Answer from the drawing. Dimensions are ordinates in mm from the lowest x, y and z of the part. Coordinates: 2 decimals unless noted, no trailing zeros. Order: outer loops, then holes, each group sorted by start corner. A loop starts at its lowest first (then second) coordinate and runs counter-clockwise, first axis right, second up. Notation, with made-up numbers: (57.25, -37.75) - (61.25, -37.75) arc R21 ccw to (61.25, -9.75) - close; hole circle Ø2 at (-4, 49). An arc over 180 degrees is marked (long way). One line per item, written item: value. Start each with the question number.
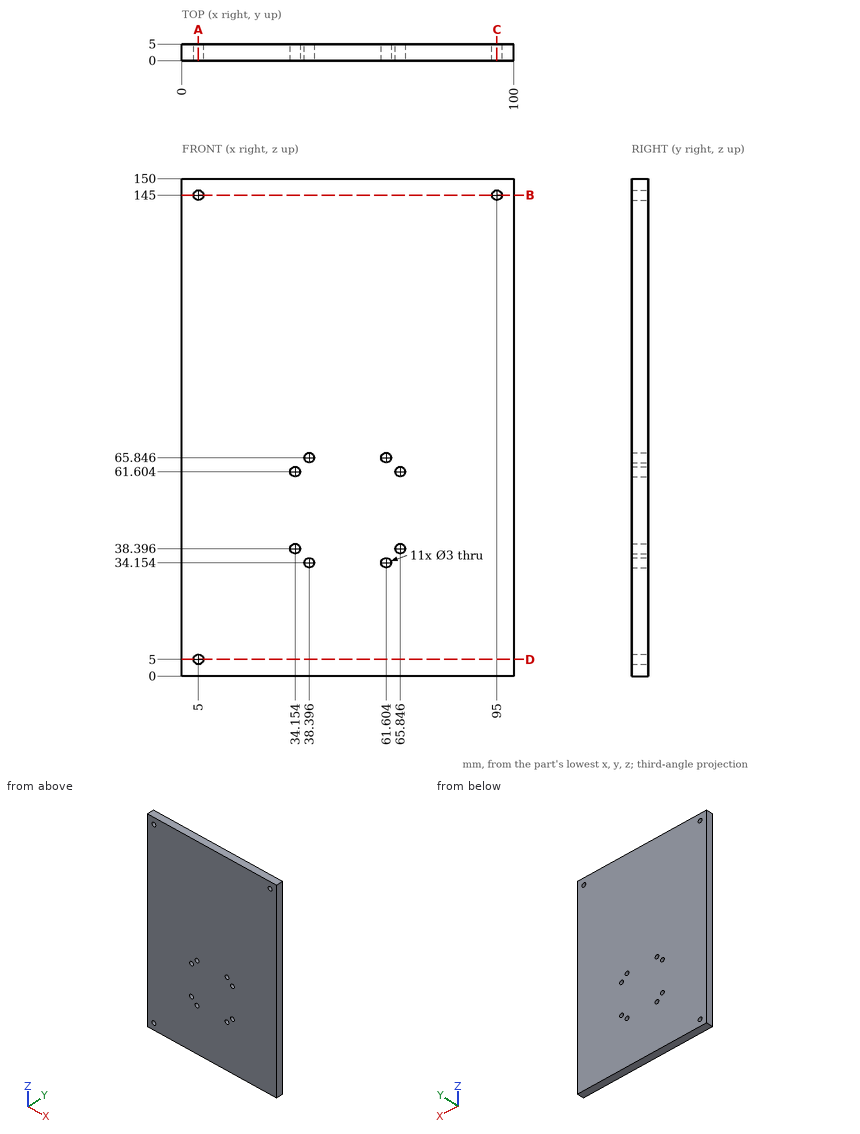
(1) Consider probe 1 along X at (y, z) = (2, 145); probe 2 along X at (y, z) = (2.9, 34) (1 decimal); probe 3 along Z at (x, y) = (5, 1.2). Determine where each line is inside the solid, lowest interval first.
(2) The part is cut by section D-D on z = 5. Determine the outline of the cut face in (x, y).
(3) The part is cut by section B-B on z = 145. Determine the outline of the cut face in (x, y), plus the area to 3 significant figures.
(4) The part is cut by section C-C on x = 95. Determine the outline of the cut face in (y, z), plus the area to 3 significant figures.
(5) The part is cut by section A-A on x = 5. Determine the outline of the cut face in (y, z).
Completed:
1. probe 1: x = 0 to 3.5, 6.5 to 93.5, 96.5 to 100
1. probe 2: x = 0 to 36.9, 39.9 to 60.1, 63.1 to 100
1. probe 3: z = 0 to 3.5, 6.5 to 143.5, 146.5 to 150
2. outline: (0, 0) - (3.5, 0) - (3.5, 5) - (0, 5) - close; (6.5, 0) - (100, 0) - (100, 5) - (6.5, 5) - close
3. outline: (0, 0) - (3.5, 0) - (3.5, 5) - (0, 5) - close; (6.5, 0) - (93.5, 0) - (93.5, 5) - (6.5, 5) - close; (96.5, 0) - (100, 0) - (100, 5) - (96.5, 5) - close
3. area: 470 mm2
4. outline: (0, 0) - (5, 0) - (5, 143.5) - (0, 143.5) - close; (0, 146.5) - (5, 146.5) - (5, 150) - (0, 150) - close
4. area: 735 mm2
5. outline: (0, 0) - (5, 0) - (5, 3.5) - (0, 3.5) - close; (0, 6.5) - (5, 6.5) - (5, 143.5) - (0, 143.5) - close; (0, 146.5) - (5, 146.5) - (5, 150) - (0, 150) - close
